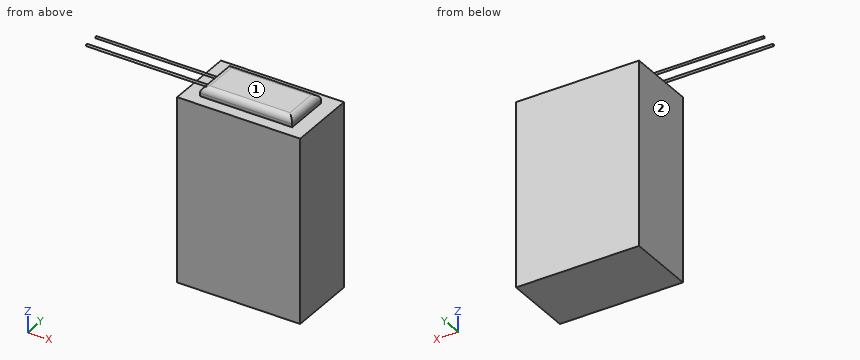
```python
from build123d import *

# Parameters (mm, degrees)
F0_W     = 50.8
F0_H     = 28.448
F1_DEPTH = 76.2
F2_W     = 38.1
F2_H     = 18.796
F3_DEPTH = 3.81
F4_R     = 2.54
F5_R     = 0.424779
F5_R_2   = 0.450135
F6_DEPTH = 50.8


with BuildPart() as f1:
    # F0 (on Top) → F1 (new body)
    with BuildSketch(Plane.XY):
        with Locations((25.4, -14.224)):
            Rectangle(F0_W, F0_H)
    extrude(amount=F1_DEPTH)

    # F2 (on face) → F3 (join)
    with BuildSketch(Plane.XY.offset(76.2)):
        with Locations((25.4, -14.224)):
            Rectangle(F2_W, F2_H)
    extrude(amount=F3_DEPTH)

    # F4
    f4_edges = [f1.edges().sort_by_distance(p)[0] for p in [
        (25.4, -4.826, 80.01),
        (25.4, -23.622, 80.01),
        (6.35, -14.224, 80.01),
        (44.45, -14.224, 80.01),
    ]]
    fillet(f4_edges, radius=F4_R)

    # F5 (on face) → F6 (join)
    with BuildSketch(Plane(origin=(6.35, 0, 0), x_dir=(0, -1, 0), z_dir=(-1, 0, 0))):
        with Locations((11.168979, 76.764129)):
            Circle(F5_R)
        with Locations((17.253665, 76.764129)):
            Circle(F5_R_2)
    extrude(amount=F6_DEPTH)


solid = f1.part
```
Geometry check sheet. Reference: the model listing, model coordinates, mm. Face numbers are marked on the shaded views. A direction names the side the tool comes from. Coordinates: 2 decimals unless noted, no trailing zeros. Order: outer loops, then holes, each group sorted by start corner. A loop starts at its lowest first (then second) coordinate and runs counter-clockwise, first axis right, second up. Notation, with made-up numbers: (-11.5, -11.5) - (18.5, -11.5) arc R28 cw to (18.5, 6.5) - close; hole circle Ø1 at (-15, 45.25). An arc over 180 degrees is marked (long way). Use one line per item in the form item = value.
1. Section check A-A (x = 29). Record the boundary of the cut face in (y, z).
Here are the results:
outline = (-28.45, 0) - (0, 0) - (0, 76.2) - (-4.83, 76.2) - (-4.83, 77.47) arc R2.54 ccw to (-7.37, 80.01) - (-21.08, 80.01) arc R2.54 ccw to (-23.62, 77.47) - (-23.62, 76.2) - (-28.45, 76.2) - close
2. Gauge pin test, flat ends, axial feed: pin 1 (0.6 mm diameter, centred on x = 16, z = 77, fed in from +Y); pin 2 (1 mm diameter, centred on x = 12, y = -6.5, fed in from +Z); pin 3 (1 mm diameter, centred on y = -18, z = 77, fed in from -X); pin 4 (8 mm diameter, centred on x = -8.5, y = -7.5, fed in from -Z). Record the tip position at first contact, or that the pin passes through.
Here are the results:
pin_1 = -4.83
pin_2 = 79.98
pin_3 = -44.45
pin_4 = 76.34
3. Section check D-D (x = -31). Record the boundary of the cut face in (y, z), then the cut area to 3 significant figures.
Here are the results:
outline = circle Ø0.9 at (-17.25, 76.76); circle Ø0.85 at (-11.17, 76.76)
area = 1.20 mm²
4. Access from +Z, -Z, +X, -X, +Y, -Y to the whole of each face (thin tool, end or side, straight path). Record for the marked faces 1 and 2.
Here are the results:
face_1 = +Z, +X, -X, +Y, -Y
face_2 = -Z, -X, +Y, -Y
5. Section check B-B (y = -19). Record the boundary of the cut face in (x, z).
Here are the results:
outline = (0, 0) - (50.8, 0) - (50.8, 76.2) - (44.45, 76.2) - (44.45, 77.47) arc R2.54 ccw to (41.91, 80.01) - (8.89, 80.01) arc R2.54 ccw to (6.35, 77.47) - (6.35, 76.2) - (0, 76.2) - close
6. Scan lines: line 1 (Z direction, x = 46, y = -11); line 2 (X direction, y = -15.5, z = 43); line 3 (Z direction, x = 32.5, y = -6.25). Record each from-to range of solid material in increasing order.
Here are the results:
line_1 = 0 to 76.2
line_2 = 0 to 50.8
line_3 = 0 to 79.75
7. Section check C-C (z = 61). Record the boundary of the cut face in (x, y), then the cut area to 3 significant figures.
Here are the results:
outline = (0, -28.45) - (50.8, -28.45) - (50.8, 0) - (0, 0) - close
area = 1,450 mm²
